Could you check a few things on this drawing? It's one solid part, dimensions in mm from its lowest x, y, z. A direction names the side the tool comes from. Coordinates: 2 decimals unless noted, no trailing zeros. Write each loop counter-clockwise with the first axis right and the second up, starting at its lowest first coordinate (ties: lowest second). Pieces come first, ordered by that corner, then holes.
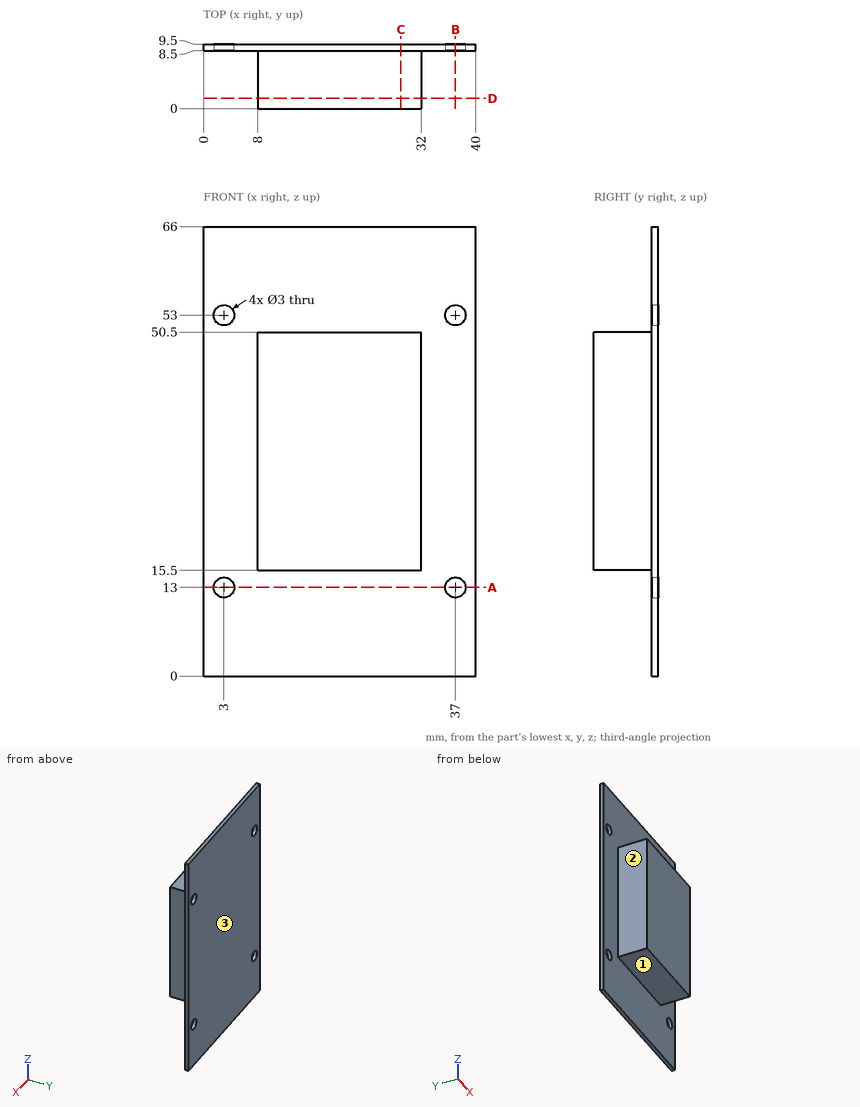
1) Imagine slicing it at A-A on z = 13. Please give me the cut outline in (x, y).
Values follow:
outline: (0, 8.5) - (1.5, 8.5) - (1.5, 9.5) - (0, 9.5) - close; (4.5, 8.5) - (35.5, 8.5) - (35.5, 9.5) - (4.5, 9.5) - close; (38.5, 8.5) - (40, 8.5) - (40, 9.5) - (38.5, 9.5) - close
2) On a 3-axis mill with a long thin cutter (end or side, diameter ignored), from which of +Z, -Z, +X, -X, +Y, -Y can I reach the whole of each face in a straight line? I mean the marked faces 1, 2 and 3. Say none if no direction works.
Values follow:
face 1: -Z, +X, -X, -Y
face 2: +Z, -Z, -X, -Y
face 3: +Z, -Z, +X, -X, +Y
3) I need wall thicknesses on probe 1 along Z at (x, y) = (37, 8.75); probe 2 along Z at (x, y) = (2, 9); probe 3 along X at (y, z) = (2.5, 27). Which ranges of each line are inside material? Lowest first, please.
Values follow:
probe 1: z = 0 to 11.5, 14.5 to 51.5, 54.5 to 66
probe 2: z = 0 to 11.88, 14.12 to 51.88, 54.12 to 66
probe 3: x = 8 to 32
4) Will these pins go through, and if not, where does the flat tip stop? pin 1 (2 mm diameter, centred on x = 11, y = 1.5, fed in from -Z); pin 2 (4 mm diameter, centred on x = 7.5, y = 4, fed in from +Z); pin 3 (1 mm diameter, centred on y = 1.5, z = 36.5, fed in from +X).
Values follow:
pin 1: stops at z = 15.5
pin 2: stops at z = 50.5
pin 3: stops at x = 32
5) Imagine slicing it at B-B on x = 37. Please give me the cut outline in (y, z), then the cut area to 3 significant figures.
Values follow:
outline: (8.5, 0) - (9.5, 0) - (9.5, 11.5) - (8.5, 11.5) - close; (8.5, 14.5) - (9.5, 14.5) - (9.5, 51.5) - (8.5, 51.5) - close; (8.5, 54.5) - (9.5, 54.5) - (9.5, 66) - (8.5, 66) - close
area: 60.0 mm2
6) Imagine slicing it at D-D on y = 1.5. Please give me the cut outline in (x, z).
Values follow:
outline: (8, 15.5) - (32, 15.5) - (32, 50.5) - (8, 50.5) - close
7) Imagine slicing it at C-C on x = 29. Please give me the cut outline in (y, z).
Values follow:
outline: (0, 15.5) - (8.5, 15.5) - (8.5, 0) - (9.5, 0) - (9.5, 66) - (8.5, 66) - (8.5, 50.5) - (0, 50.5) - close
